Check sheet for the modelled part. Datum: model origin and axes. Units: mm. A direction names the side the tool comes from. Coordinates: 2 decimals unless noted, no trailing zeros. Loops run counter-clockwise (first coordinate to the right, second up) from the corner with the lowest first, then second, coordinate; pieces in that order, holes last. Notation, with made-up numbers: (66.25, -18.75) - (122.25, -18.75) arc R15 ccw to (122.25, -12.75) - close; hole circle Ø11 at (-32.5, -7.5). An arc over 180 degrees is marked (long way). Use a Markdown table: item, result. Add a question column.
1) Sectioned sample at D-D, the plane x = 11. Enter the section's corners in (y, z).
2) Tool access check on faces 1 (the cylindrical face through (10.97, 0.99, -38.1)), 2 (the cylindrical face through (-21.49, 1.51, -8.6)). Record the directions out of +Z, -Z, +X, -X, +Y, -Y that give a thin tool (end or side, any length) a straight path to the whole face; none if there is none.
3) Sectioned sample at C-C, the plane x = -24.26. Enter the section's corners in (y, z).
4) Sectioned sample at B-B, the plane y = 0.45. State how many separate pieces and enclosed holes the cut face has, then the cut area to 3 significant figures.
5) Go/stop test with a flat-tipped pin: P1, Ø13, axis at x = -12.7, z = 42.64, coming from the +Y side. Record where the tip stops, or that it passes through.
6) Thickness scan on line 1 (Z direction, x = -12.7, y = 0.85); line 2 (X direction, y = 1, z = 17.63); line 3 (X direction, y = 1.35, z = -19.75). Record the ranges inside material, lowest first.
7) Draft check along X on faces 3 (the cylindrical face through (-25.734, 0.493, -11.102)), 4 (the cylindrical face through (-27.93, 0.99, 58.1)), 5 (the flat face through (0, 0, -1)). Enter one of: pulls with the +X half, pulls with the -X half, needs draft (parallel to the pull), parting line crosses it, or undercut.
8) Sectioned sample at A-A, the plane z = -9.75. Enter the section's corners in (x, y), then the cut area to 3 significant figures.
from build123d import *

# Parameters (mm, degrees)
SKETCH1_R           = 8
SKETCH1_R_2         = 2
BOSS_EXTRUDE1_DEPTH = 2
SKETCH2_R           = 3
CUT_EXTRUDE1_DEPTH  = 1


with BuildPart() as part:
    # Sketch1 → Boss-Extrude1 (new body)
    with BuildSketch(Plane(origin=(0, 0, 0), x_dir=(1, 0, 0), z_dir=(0, 1, 0))):
        with BuildLine():
            Line((19.05, -61.72), (-19.05, -61.72))
            ThreePointArc((-19.05, -61.72), (-28.030256121, -58.000256121), (-31.75, -49.02))
            Line((-31.75, -49.02), (-31.75, 49.02))
            ThreePointArc((-31.75, 49.02), (-28.030256121, 58.000256121), (-19.05, 61.72))
            Line((-19.05, 61.72), (19.05, 61.72))
            ThreePointArc((19.05, 61.72), (28.030256121, 58.000256121), (31.75, 49.02))
            Line((31.75, 49.02), (31.75, -49.02))
            ThreePointArc((31.75, -49.02), (28.030256121, -58.000256121), (19.05, -61.72))
        make_face()
        with Locations((-12.7, 45.91)):
            Circle(SKETCH1_R, mode=Mode.SUBTRACT)
        with Locations((12.7, 45.91)):
            Circle(SKETCH1_R, mode=Mode.SUBTRACT)
        with Locations((-12.7, -42.64)):
            Circle(SKETCH1_R, mode=Mode.SUBTRACT)
        with Locations((12.7, -42.64)):
            Circle(SKETCH1_R, mode=Mode.SUBTRACT)
        with Locations((12.7, -17.63)):
            Circle(SKETCH1_R, mode=Mode.SUBTRACT)
        with Locations((-12.7, -17.63)):
            Circle(SKETCH1_R, mode=Mode.SUBTRACT)
        with Locations((-24.26, 19.75)):
            Circle(SKETCH1_R_2, mode=Mode.SUBTRACT)
        with Locations((-24.26, 9.75)):
            Circle(SKETCH1_R_2, mode=Mode.SUBTRACT)
        with Locations((24.26, 19.75)):
            Circle(SKETCH1_R_2, mode=Mode.SUBTRACT)
        with Locations((24.26, 9.75)):
            Circle(SKETCH1_R_2, mode=Mode.SUBTRACT)
    extrude(amount=BOSS_EXTRUDE1_DEPTH)

    # Sketch2 → Cut-Extrude1 (cut)
    with BuildSketch(Plane(origin=(0, 2, 0), x_dir=(1, 0, 0), z_dir=(0, 1, 0))):
        with Locations((-24.26, 19.75)):
            Circle(SKETCH2_R)
        with Locations((-24.26, 9.75)):
            Circle(SKETCH2_R)
        with Locations((24.26, 19.75)):
            Circle(SKETCH2_R)
        with Locations((24.26, 9.75)):
            Circle(SKETCH2_R)
    extrude(amount=-CUT_EXTRUDE1_DEPTH, mode=Mode.SUBTRACT)


solid = part.part
Solved:
| question | item | result |
|---|---|---|
| 1 | outline | (0, -61.72) - (2, -61.72) - (2, -53.73) - (0, -53.73) - close; (0, -38.09) - (2, -38.09) - (2, 9.81) - (0, 9.81) - close; (0, 25.45) - (2, 25.45) - (2, 34.82) - (0, 34.82) - close; (0, 50.46) - (2, 50.46) - (2, 61.72) - (0, 61.72) - close |
| 2 | face 1 | +Y, -Y |
| 2 | face 2 | +Y |
| 3 | outline | (0, -60.6) - (2, -60.6) - (2, -22.75) - (1, -22.75) - (1, -21.75) - (0, -21.75) - close; (0, -17.75) - (1, -17.75) - (1, -16.75) - (2, -16.75) - (2, -12.75) - (1, -12.75) - (1, -11.75) - (0, -11.75) - close; (0, -7.75) - (1, -7.75) - (1, -6.75) - (2, -6.75) - (2, 60.6) - (0, 60.6) - close |
| 4 | separate pieces | 1 |
| 4 | enclosed holes | 10 |
| 4 | area | 6,440 mm2 |
| 5 | P1 | passes through |
| 6 | line 1 | z = -61.72 to -53.91, -37.91 to 9.63, 25.63 to 34.64, 50.64 to 61.72 |
| 6 | line 2 | x = -31.75 to -20.7, -4.7 to 4.7, 20.7 to 31.75 |
| 6 | line 3 | x = -31.75 to -27.26, -21.26 to 21.26, 27.26 to 31.75 |
| 7 | face 3 | undercut |
| 7 | face 4 | pulls with the -X half |
| 7 | face 5 | needs draft |
| 8 | outline | (-31.75, 0) - (-26.26, 0) - (-26.26, 1) - (-27.26, 1) - (-27.26, 2) - (-31.75, 2) - close; (-22.26, 0) - (22.26, 0) - (22.26, 1) - (21.26, 1) - (21.26, 2) - (-21.26, 2) - (-21.26, 1) - (-22.26, 1) - close; (26.26, 0) - (31.75, 0) - (31.75, 2) - (27.26, 2) - (27.26, 1) - (26.26, 1) - close |
| 8 | area | 107 mm2 |
